Can you work these out from the model? Positions are in its coordinate system, mm. Coordinates: 2 decimals unless noted, no trailing zeros. Order: outer loops, then holes, each group sorted by start corner. A loop starts at its lowest first (then second) coordinate and runs counter-clockwise, first axis right, second up. Notation, with made-up numbers: (80.5, 31.5) -> (108.5, 31.5) arc R18 cw to (108.5, 50.5) -> close; hole circle Ø6 at (16, -2.75). An arc over 180 degrees is marked (long way). Answer in a Markdown table with one row per item.
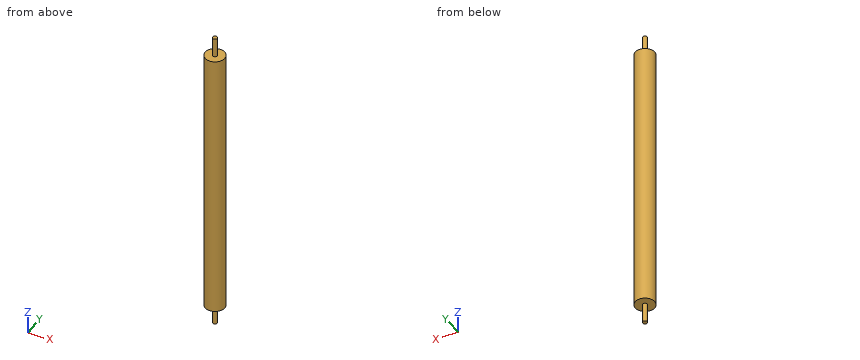
```python
from build123d import *

# Parameters (mm, degrees)
F0_R     = 63.5
F1_DEPTH = 1803.4
F3_R     = 15.24
F4_DEPTH = 127
F5_R     = 15.24
F6_DEPTH = 127


with BuildPart() as f1:
    # F0 (on Top) → F1 (new body)
    with BuildSketch(Plane.XY):
        Circle(F0_R)
    extrude(amount=F1_DEPTH)

    # F3 (on offset) → F4 (join)
    with BuildSketch(Plane.XY.offset(1803.4)):
        Circle(F3_R)
    extrude(amount=F4_DEPTH)

    # F5 (on Top) → F6 (join)
    with BuildSketch(Plane.XY):
        Circle(F5_R)
    extrude(amount=-F6_DEPTH)


solid = f1.part
```
(1) Suppose I cut it at C-C (y = -34.5). Please give me the cut outline in (x, z).
Response values:
| item | result |
|---|---|
| outline | (-53.31, 0) -> (53.31, 0) -> (53.31, 1803.4) -> (-53.31, 1803.4) -> close |
(2) Will these pins go through, and if not, where does the flat tip stop? pin 1 Ø8 at (y, z) = (-23.5, 384) entering from -X; pin 2 Ø1.5 at (x, z) = (13.5, 1133.5) entering from -Y; pin 3 Ø4 at (x, z) = (-15.5, 1600) entering from -Y.
Response values:
| item | result |
|---|---|
| pin 1 | x = -60.43 |
| pin 2 | y = -62.21 |
| pin 3 | y = -62.05 |
(3) Suppose I cut it at A-A (x = -32). Please give me the cut outline in (y, z), and give its area (3 significant figures).
Response values:
| item | result |
|---|---|
| outline | (-54.85, 0) -> (54.85, 0) -> (54.85, 1803.4) -> (-54.85, 1803.4) -> close |
| area | 198,000 mm2 |
(4) Suppose I cut it at B-B (z = 303). Please give me the cut outline in (x, y), and give its area (3 significant figures).
Response values:
| item | result |
|---|---|
| outline | circle Ø127 at (0, 0) |
| area | 12,700 mm2 |
(5) I need wall thicknesses on line 1 (Z direction, x = -34.5, y = 11.5); line 2 (Y direction, x = -1.5, z = 1606); line 3 (Y direction, x = -54, z = 198.5). Which ranges of each line are inside material? Lowest first, please. Write a range as [from, to].
Response values:
| item | result |
|---|---|
| line 1 | [0, 1803.4] |
| line 2 | [-63.48, 63.48] |
| line 3 | [-33.41, 33.41] |
